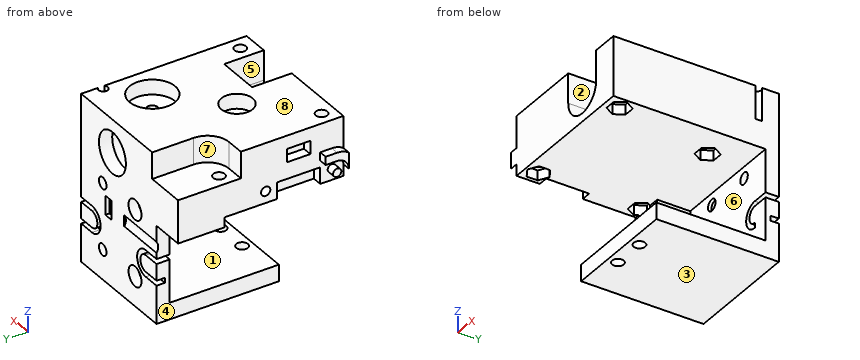
from build123d import *

# Parameters (mm, degrees)
SKETCH1_W                = 35
SKETCH1_H                = 28
BOSS_EXTRUDE1_DEPTH      = 4
SKETCH2_R                = 1.75
CUT_EXTRUDE1_DEPTH       = 23.765104876
BOSS_EXTRUDE2_DEPTH      = 17.5
BOSS_EXTRUDE2_DEPTH_BACK = 0.5
SKETCH3_W                = 35
SKETCH3_H                = 50
SKETCH7_W                = 35
SKETCH7_H                = 37
BOSS_EXTRUDE3_DEPTH      = 5
SKETCH10_R               = 1.75
CUT_EXTRUDE6_DEPTH       = 5
SKETCH24_W               = 18
SKETCH24_H               = 46
BOSS_EXTRUDE4_DEPTH      = 10
SKETCH37_W               = 13
SKETCH37_H               = 14
BOSS_EXTRUDE9_DEPTH      = 10
CUT_EXTRUDE19_REACH      = 75.638
SKETCH22_R               = 1.75
SKETCH22_3_R             = 6.9
SKETCH22_3_R_2           = 4.75
CUT_EXTRUDE20_DEPTH      = 4.5
SKETCH22_5_R             = 1.75
SKETCH22_5_W             = 2
SKETCH22_5_H             = 4
CUT_EXTRUDE24_DEPTH      = 8
SKETCH22_4_W             = 13
SKETCH22_4_H             = 12
CUT_EXTRUDE21_DEPTH      = 15.5
FILLET3_R                = 6.5
SKETCH26_R               = 2.25
CUT_EXTRUDE22_DEPTH      = 57.502212346
SKETCH27_R               = 6.25
CUT_EXTRUDE23_DEPTH      = 8
CUT_EXTRUDE25_DEPTH      = 3
CUT_EXTRUDE25_DEPTH_BACK = 3
SKETCH30_R               = 3
CUT_EXTRUDE26_DEPTH      = 3
CUT_EXTRUDE27_DEPTH      = 66.180518562
SKETCH32_W               = 5
SKETCH32_H               = 1.5
CUT_EXTRUDE28_DEPTH      = 2.5
SKETCH33_R               = 3
CUT_EXTRUDE29_DEPTH      = 15
SKETCH34_W               = 2.8
SKETCH34_H               = 5.8
CUT_EXTRUDE30_DEPTH      = 1.2
SKETCH38_R               = 7
CUT_EXTRUDE31_DEPTH      = 4
SKETCH39_W               = 5
SKETCH39_H               = 13
SKETCH39_W_2             = 4
SKETCH39_H_2             = 7
CUT_EXTRUDE32_DEPTH      = 3
SKETCH40_R               = 1.4
CUT_EXTRUDE33_DEPTH      = 15
SKETCH41_R               = 1.25
BOSS_EXTRUDE10_DEPTH     = 2.5
SKETCH42_R               = 1.4
CUT_EXTRUDE34_DEPTH      = 10


with BuildPart() as part:
    # Sketch1 → Boss-Extrude1 (new body)
    with BuildSketch(Plane(origin=(0, 0, 0), x_dir=(1, 0, 0), z_dir=(0, 1, 0))):
        Rectangle(SKETCH1_W, SKETCH1_H)
    extrude(amount=BOSS_EXTRUDE1_DEPTH)

    # Sketch2 → Cut-Extrude1 (cut, through all)
    with BuildSketch(Plane(origin=(0, 4, 0), x_dir=(1, 0, 0), z_dir=(0, 1, 0))):
        with Locations(Location((-7.5, -10, 0), (0, 0, 270))):
            Circle(SKETCH2_R)
        with Locations(Location((-7.5, 10, 0), (0, 0, 270))):
            Circle(SKETCH2_R)
        with Locations(Location((7.5, -10, 0), (0, 0, 270))):
            Circle(SKETCH2_R)
        with Locations(Location((7.5, 10, 0), (0, 0, 270))):
            Circle(SKETCH2_R)
    extrude(amount=-CUT_EXTRUDE1_DEPTH, mode=Mode.SUBTRACT)

    # Sketch3 → Boss-Extrude2 (add, two sides: drawn at the far end of the back side and taken through both)
    with BuildSketch(Plane.XY.offset(14).offset(-BOSS_EXTRUDE2_DEPTH_BACK)):
        with Locations((0, -21)):
            Rectangle(SKETCH3_W, SKETCH3_H)
    extrude(amount=BOSS_EXTRUDE2_DEPTH + BOSS_EXTRUDE2_DEPTH_BACK)

    # Sketch7 → Boss-Extrude3 (add)
    with BuildSketch(Plane(origin=(0, 0, -14), x_dir=(-1, 0, 0), z_dir=(0, 0, -1))):
        with Locations((0, -14.5)):
            Rectangle(SKETCH7_W, SKETCH7_H)
    extrude(amount=BOSS_EXTRUDE3_DEPTH)

    # Sketch10 → Cut-Extrude6 (cut)
    with BuildSketch(Plane(origin=(0, 0, -19), x_dir=(-1, 0, 0), z_dir=(0, 0, -1))):
        with Locations((-5, -30)):
            Circle(SKETCH10_R)
        with Locations((5, -30)):
            Circle(SKETCH10_R)
    extrude(amount=-CUT_EXTRUDE6_DEPTH, mode=Mode.SUBTRACT)

    # Sketch24 → Boss-Extrude4 (add)
    with BuildSketch(Plane.ZY.offset(17.5)):
        with Locations((22.5, -23)):
            Rectangle(SKETCH24_W, SKETCH24_H)
    extrude(amount=BOSS_EXTRUDE4_DEPTH)

    # Sketch37 → Boss-Extrude9 (add)
    with BuildSketch(Plane.ZY.offset(17.5)):
        with Locations((17, -3)):
            Rectangle(SKETCH37_W, SKETCH37_H)
    extrude(amount=BOSS_EXTRUDE9_DEPTH)

    # Sketch22 → Cut-Extrude19 (cut, up to next)
    with BuildSketch(Plane.XY.offset(31.5), mode=Mode.PRIVATE) as cut_extrude19_sk1:
        with Locations((-23.5, -42)):
            Circle(SKETCH22_R)
    cut_extrude19_tool1 = extrude(cut_extrude19_sk1.sketch, amount=-CUT_EXTRUDE19_REACH, mode=Mode.PRIVATE) & part.part
    # Sketch22 → Cut-Extrude19 (cut, up to next)
    with BuildSketch(Plane.XY.offset(31.5), mode=Mode.PRIVATE) as cut_extrude19_sk2:
        with Locations((13.5, -41.5)):
            Circle(SKETCH22_R)
    cut_extrude19_tool2 = extrude(cut_extrude19_sk2.sketch, amount=-CUT_EXTRUDE19_REACH, mode=Mode.PRIVATE) & part.part
    # Sketch22 → Cut-Extrude19 (cut, up to next)
    with BuildSketch(Plane.XY.offset(31.5), mode=Mode.PRIVATE) as cut_extrude19_sk3:
        with Locations((7.5, -11)):
            Circle(SKETCH22_R)
    cut_extrude19_tool3 = extrude(cut_extrude19_sk3.sketch, amount=-CUT_EXTRUDE19_REACH, mode=Mode.PRIVATE) & part.part
    # Sketch22 → Cut-Extrude19 (cut, up to next)
    with BuildSketch(Plane.XY.offset(31.5), mode=Mode.PRIVATE) as cut_extrude19_sk4:
        with Locations((-23.5, -11)):
            Circle(SKETCH22_R)
    cut_extrude19_tool4 = extrude(cut_extrude19_sk4.sketch, amount=-CUT_EXTRUDE19_REACH, mode=Mode.PRIVATE) & part.part
    add(cut_extrude19_tool1.solids().sort_by_distance((-23.5, -42, 31.5))[0], mode=Mode.SUBTRACT)
    add(cut_extrude19_tool2.solids().sort_by_distance((13.5, -41.5, 31.5))[0], mode=Mode.SUBTRACT)
    add(cut_extrude19_tool3.solids().sort_by_distance((7.5, -11, 31.5))[0], mode=Mode.SUBTRACT)
    add(cut_extrude19_tool4.solids().sort_by_distance((-23.5, -11, 31.5))[0], mode=Mode.SUBTRACT)

    # Sketch22<3> → Cut-Extrude20 (cut)
    with BuildSketch(Plane.XY.offset(31.5)):
        with Locations((7.5, -11)):
            Circle(SKETCH22_3_R)
        with Locations((-8, -26.5)):
            Circle(SKETCH22_3_R_2)
    extrude(amount=-CUT_EXTRUDE20_DEPTH, mode=Mode.SUBTRACT)

    # Sketch22<5> → Cut-Extrude24 (cut)
    # profile 1 of 2: a face of its own
    with BuildSketch(Plane.XY.offset(31.5)):
        with BuildLine():
            Line((-15.5, -8.5), (-15.5, 0))
            Line((-15.5, 0), (-17.5, 0))
            Line((-17.5, 0), (-27.5, 0))
            Line((-27.5, 0), (-27.5, -15))
            Line((-27.5, -15), (-22, -15))
            ThreePointArc((-22, -15), (-17.403805922, -13.096194078), (-15.5, -8.5))
        make_face()
        with Locations((-23.5, -11)):
            Circle(SKETCH22_5_R, mode=Mode.SUBTRACT)
    # profile 2 of 2: a face of its own
    with BuildSketch(Plane.XY.offset(31.5)):
        with Locations((-16.5, 2)):
            Rectangle(SKETCH22_5_W, SKETCH22_5_H)
    extrude(amount=-CUT_EXTRUDE24_DEPTH, mode=Mode.SUBTRACT)

    # Sketch22<4> → Cut-Extrude21 (cut)
    with BuildSketch(Plane.XY.offset(31.5)):
        with Locations((3, -40)):
            Rectangle(SKETCH22_4_W, SKETCH22_4_H)
    extrude(amount=-CUT_EXTRUDE21_DEPTH, mode=Mode.SUBTRACT)

    # Fillet3
    fillet3_edges = [part.edges().sort_by_distance(p)[0] for p in [
        (9.5, -40, 16),
        (-3.5, -40, 16),
    ]]
    fillet(fillet3_edges, radius=FILLET3_R - 0.0001)  # a hair under: the kernel refuses the full size

    # Sketch26 → Cut-Extrude22 (cut, through all)
    with BuildSketch(Plane.XZ.offset(34)):
        with Locations(Location((3, 21.5, 0), (0, 0, 270))):
            Circle(SKETCH26_R)
    extrude(amount=-CUT_EXTRUDE22_DEPTH, mode=Mode.SUBTRACT)

    # Sketch27 → Cut-Extrude23 (cut)
    with BuildSketch(Plane(origin=(0, 4, 0), x_dir=(1, 0, 0), z_dir=(0, 1, 0))):
        with Locations(Location((3, -21.5, 0), (0, 0, 270))):
            Circle(SKETCH27_R)
    extrude(amount=-CUT_EXTRUDE23_DEPTH, mode=Mode.SUBTRACT)

    # Sketch29 → Cut-Extrude25 (cut, two sides: drawn at the far end of the back side and taken through both)
    with BuildSketch(Plane(origin=(0, 0, 13.5), x_dir=(-1, 0, 0), z_dir=(0, 0, -1)).offset(-CUT_EXTRUDE25_DEPTH_BACK)):
        Polygon((-4.151368439, -11), (-5.825684219, -8.1), (-9.174315781, -8.1), (-10.848631561, -11), (-9.174315781, -13.9), (-5.825684219, -13.9), align=None)
        Polygon((20.151368439, -11), (21.825684219, -13.9), (25.174315781, -13.9), (26.848631561, -11), (25.174315781, -8.1), (21.825684219, -8.1), align=None)
        Polygon((-10.151368439, -41.5), (-11.825684219, -38.6), (-15.174315781, -38.6), (-16.848631561, -41.5), (-15.174315781, -44.4), (-11.825684219, -44.4), align=None)
        Polygon((23.5, -45.348631561), (26.4, -43.674315781), (26.4, -40.325684219), (23.5, -38.651368439), (20.6, -40.325684219), (20.6, -43.674315781), align=None)
    extrude(amount=CUT_EXTRUDE25_DEPTH + CUT_EXTRUDE25_DEPTH_BACK, mode=Mode.SUBTRACT)

    # Sketch30 → Cut-Extrude26 (cut)
    with BuildSketch(Plane(origin=(0, 4, 0), x_dir=(1, 0, 0), z_dir=(0, 1, 0))):
        with Locations(Location((-7.5, 10, 0), (0, 0, 270))):
            Circle(SKETCH30_R)
        with Locations(Location((-7.5, -10, 0), (0, 0, 270))):
            Circle(SKETCH30_R)
    extrude(amount=-CUT_EXTRUDE26_DEPTH, mode=Mode.SUBTRACT)

    # Sketch31 → Cut-Extrude27 (cut, through all)
    with BuildSketch(Plane(origin=(0, 4, 0), x_dir=(1, 0, 0), z_dir=(0, 1, 0))):
        with BuildLine():
            Line((-17.5, 1), (-12.5, 1))
            ThreePointArc((-12.5, 1), (-10, 3.5), (-12.5, 6))
            Line((-12.5, 6), (-12.5, 7.5))
            ThreePointArc((-12.5, 7.5), (-8.5, 3.5), (-12.5, -0.5))
            Line((-12.5, -0.5), (-17.5, -0.5))
            Line((-17.5, -0.5), (-17.5, 1))
        make_face()
    cut_extrude27 = extrude(amount=-CUT_EXTRUDE27_DEPTH, mode=Mode.SUBTRACT)

    # Sketch32 → Cut-Extrude28 (cut)
    with BuildSketch(Plane(origin=(0, 4, 0), x_dir=(1, 0, 0), z_dir=(0, 1, 0))):
        with Locations((-15, 6.75)):
            Rectangle(SKETCH32_W, SKETCH32_H)
    cut_extrude28 = extrude(amount=-CUT_EXTRUDE28_DEPTH, mode=Mode.SUBTRACT)

    # Sketch33 → Cut-Extrude29 (cut)
    with BuildSketch(Plane.ZY.offset(17.5)):
        with Locations((4, 6.5)):
            Circle(SKETCH33_R)
    extrude(amount=-CUT_EXTRUDE29_DEPTH, mode=Mode.SUBTRACT)

    # Sketch34 → Cut-Extrude30 (cut)
    with BuildSketch(Plane(origin=(0, 4, 0), x_dir=(1, 0, 0), z_dir=(0, 1, 0))):
        with Locations((4.9, -4)):
            Rectangle(SKETCH34_W, SKETCH34_H)
    extrude(amount=-CUT_EXTRUDE30_DEPTH, mode=Mode.SUBTRACT)

    # Mirror1: Cut-Extrude27, Cut-Extrude28 across plane
    add(cut_extrude27.mirror(Plane.ZY), mode=Mode.SUBTRACT)
    add(cut_extrude28.mirror(Plane.ZY), mode=Mode.SUBTRACT)

    # Sketch38 → Cut-Extrude31 (cut)
    with BuildSketch(Plane(origin=(0, -4, 0), x_dir=(1, 0, 0), z_dir=(0, 1, 0))):
        with Locations(Location((3, -21.5, 0), (0, 0, 270))):
            Circle(SKETCH38_R)
    extrude(amount=CUT_EXTRUDE31_DEPTH, mode=Mode.SUBTRACT)

    # Sketch39 → Cut-Extrude32 (cut)
    with BuildSketch(Plane.ZY.offset(27.5)):
        with Locations((16, -32.5)):
            Rectangle(SKETCH39_W, SKETCH39_H)
        with Locations((25.5, -32.5)):
            Rectangle(SKETCH39_W_2, SKETCH39_H_2)
    extrude(amount=-CUT_EXTRUDE32_DEPTH, mode=Mode.SUBTRACT)

    # Sketch40 → Cut-Extrude33 (cut)
    with BuildSketch(Plane.ZY.offset(27.5)):
        with Locations((17, -22.5)):
            Circle(SKETCH40_R)
    extrude(amount=-CUT_EXTRUDE33_DEPTH, mode=Mode.SUBTRACT)

    # Sketch41 → Boss-Extrude10 (add)
    with BuildSketch(Plane.ZY.offset(27.5)):
        with Locations(Location((17, -42.5, 0), (0, 0, 180))):
            Circle(SKETCH41_R)
        with BuildLine():
            Line((20.5, -39), (20.5, -42.5))
            ThreePointArc((20.5, -42.5), (19.474873734, -44.974873734), (17, -46))
            Line((17, -46), (21.873397172, -46))
            ThreePointArc((21.873397172, -46), (22.711408891, -44.338425545), (23, -42.5))
            Line((23, -42.5), (23, -39))
            Line((23, -39), (20.5, -39))
        make_face()
    extrude(amount=BOSS_EXTRUDE10_DEPTH)

    # Sketch42 → Cut-Extrude34 (cut)
    with BuildSketch(Plane.XY.offset(31.5)):
        with Locations((16.5, -2)):
            Circle(SKETCH42_R)
    extrude(amount=-CUT_EXTRUDE34_DEPTH, mode=Mode.SUBTRACT)


solid = part.part
The listing builds one solid part. Answer for the finished solid, in the listing's coordinates (mm). Face numbers are marked on the shaded views. A direction names the side the tool comes from. Give positions to 0.01 mm unless a question says otherwise; leave off trailing zeros. Write each loop counter-clockwise with the first axis right and the second up, starting at its lowest first coordinate (ties: lowest second). Pieces come first, ordered by that corner, then holes. Notation, with made-up numbers: (-26.75, -12) -> (3.25, -12) arc R31 ccw to (3.25, 13) -> close; hole circle Ø1 at (83.5, 86.5). An arc over 180 degrees is marked (long way). Use a Markdown table: item, result.
(1) Find the intervals of material crossed by probe 1 along Y at (x, z) = (-23.5, 22); probe 2 along X at (y, z) = (1.55, -10); probe 3 along Y at (x, z) = (-25.5, 24), in increasing order. Write a range as from..to.
Return value:
| item | result |
|---|---|
| probe 1 | -46..-43.75, -40.25..-12.75, -9.25..4 |
| probe 2 | -17.5..-10.5, -4.5..5.75, 9.25..17.5 |
| probe 3 | -46..-36, -29..-15 |
(2) Flat-ended cylindrical pins translate along their axes: P1, Ø3, axis at x = -23, y = -43, coming from the -Z side; P2, Ø6.5, axis at y = -23, z = 19.5, coming from the -X side; P3, Ø8, axis at y = -21.5, z = -14, coming from the -X side. Find the tip coordinate at first contact, or state that the pin passes through.
Return value:
| item | result |
|---|---|
| P1 | z = 16.5 |
| P2 | x = -27.5 |
| P3 | x = -17.5 |
(3) Section C-C, the plane z = 25 is taken. Determine the outline of the cut face in (x, y).
Return value:
| item | result |
|---|---|
| outline | (-27.5, -46) -> (-3.5, -46) -> (-3.5, -34) -> (9.5, -34) -> (9.5, -46) -> (17.5, -46) -> (17.5, -2.98) arc R1.4 cw (long way) to (17.5, -1.02) -> (17.5, 4) -> (8.18, 4) -> (8.18, 0) -> (9.06, 0) -> (9.06, -4) -> (-3.06, -4) -> (-3.06, 0) -> (-2.18, 0) -> (-2.18, 4) -> (-15.5, 4) -> (-15.5, -8.5) arc R6.5 cw to (-22, -15) -> (-27.5, -15) -> (-27.5, -29) -> (-24.5, -29) -> (-24.5, -36) -> (-27.5, -36) -> close; hole circle Ø3.5 at (-23.5, -42); hole circle Ø3.5 at (7.5, -11); hole circle Ø3.5 at (13.5, -41.5) |
(4) Determine the mould class of the marked faces 1, 2 and 3 for opening direction Z: released by +Z, released by -Z, zero draft, split by the parting line, or undercut.
Return value:
| item | result |
|---|---|
| face 1 | undercut |
| face 2 | zero draft |
| face 3 | released by -Z |
(5) Section B-B, the plane y = -30 is taken. Determine the outline of the cut face in (x, z).
Return value:
| item | result |
|---|---|
| outline | (-27.5, 18.5) -> (-24.5, 18.5) -> (-24.5, 13.5) -> (17.5, 13.5) -> (17.5, 31.5) -> (-4.79, 31.5) -> (-4.79, 27) -> (-11.21, 27) -> (-11.21, 31.5) -> (-27.5, 31.5) -> (-27.5, 27.5) -> (-24.5, 27.5) -> (-24.5, 23.5) -> (-27.5, 23.5) -> close; (-17.5, -19) -> (-6.75, -19) -> (-6.75, -14) -> (-17.5, -14) -> close; (-3.25, -19) -> (3.25, -19) -> (3.25, -14) -> (-3.25, -14) -> close; (6.75, -19) -> (17.5, -19) -> (17.5, -14) -> (6.75, -14) -> close; hole circle Ø4.5 at (3, 21.5) |
(6) For the marked faces 4, 5, 6, 7 and 8, determine the directions among +Z, -Z, +X, -X, +Y, -Y from which every point of the face is accessible in a straight line to the end or side of a thin tool.
Return value:
| item | result |
|---|---|
| face 4 | -Z, -X, +Y, -Y |
| face 5 | +Z, -Y |
| face 6 | +X, -Y |
| face 7 | +Z, -X, +Y |
| face 8 | +Z, +X, -X, +Y, -Y |
(7) Section A-A, the plane z = -3.5 is taken. Determine the outline of the cut face in (x, y).
Return value:
| item | result |
|---|---|
| outline | (-17.5, 0) -> (-10, 0) -> (-10, 4) -> (-17.5, 4) -> close; (-8.5, 0) -> (8.5, 0) -> (8.5, 4) -> (-8.5, 4) -> close; (10, 0) -> (17.5, 0) -> (17.5, 4) -> (10, 4) -> close |
